Print and shaded views of the part. All mm, measured from the part's lowest x, y and z. A direction names the side the tool comes from. Round coordinates to 2 decimals unless told otherwise and drop trailing zeros. Loops run counter-clockwise (first coordinate to the right, second up) from the corner with the lowest first, then second, coordinate; pieces in that order, holes last. Notation, with made-up numbers: (54, -16.5) -> (105, -16.5) arc R20 ccw to (105, -2.5) -> close; hole circle Ø8 at (-27, 69). An arc over 180 degrees is marked (long way). Answer as CSV lines item,"result".
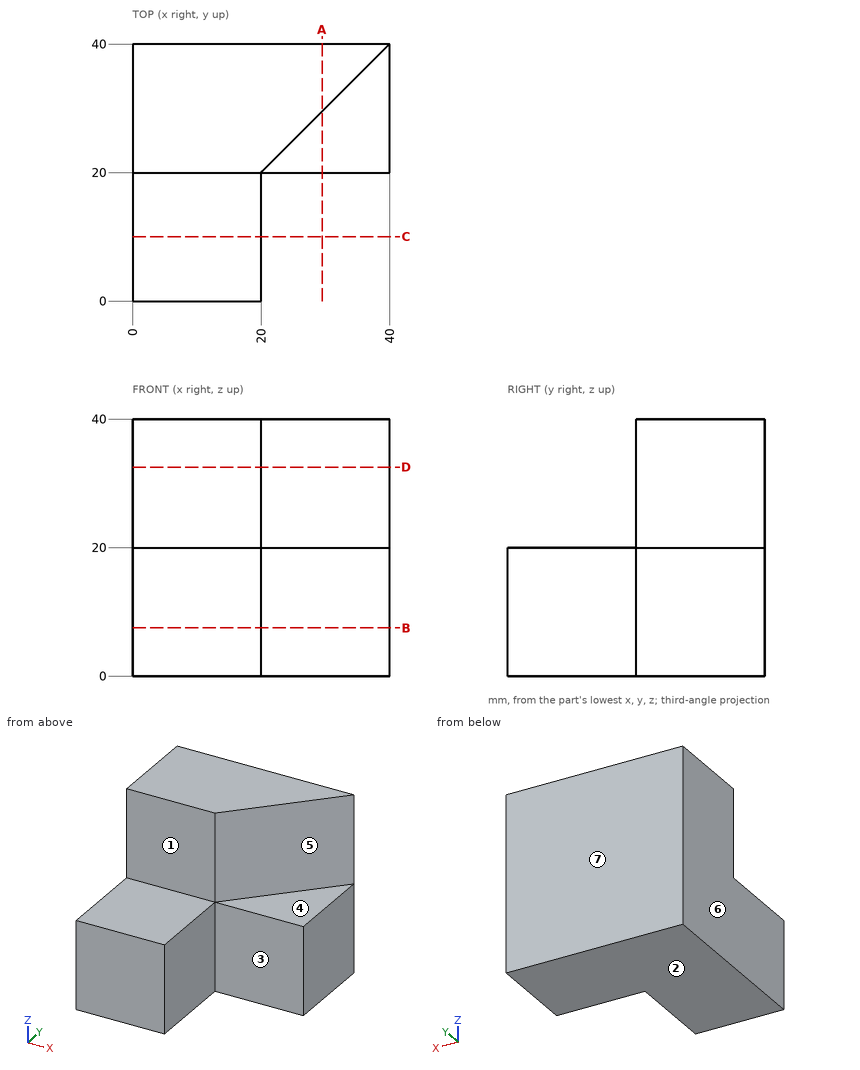
Q1. Saw through at D-D, the plane z = 32.5. Write the cut outline in (x, y).
Geometry results:
outline,"(0, 20) -> (20, 20) -> (40, 40) -> (0, 40) -> close"
Q2. Saw through at C-C, the plane y = 10. Write the cut outline in (x, z).
Geometry results:
outline,"(0, 0) -> (20, 0) -> (20, 20) -> (0, 20) -> close"
Q3. Saw through at A-A, the plane x = 29.5. Write the cut outline in (y, z).
Geometry results:
outline,"(20, 0) -> (40, 0) -> (40, 40) -> (29.5, 40) -> (29.5, 20) -> (20, 20) -> close"
Q4. Which spindle directions (+Z, -Z, +X, -X, +Y, -Y) get a long thin tool onto all of the face, cutting with end or side? Do the marked faces 1, 2, 3 and 4. Say none if no direction does.
Geometry results:
face 1,"+Z, +X, -X, -Y"
face 2,"-Z, +X, -X, +Y, -Y"
face 3,"+Z, -Z, +X, -Y"
face 4,"+Z, +X, -Y"
Q5. Drop flat-ended pins along their axis: P1, Ø10, axis at x = 5.5, z = 34.5, coming from the -Y side; P2, Ø12, axis at y = 22.5, z = 24, coming from the -X side; P3, Ø10, axis at x = 8.5, y = 5, coming from the +Z side; P4, Ø1, axis at y = 17.5, z = 11, coming from the +X side. Give the stop position or say it passes through.
Geometry results:
P1,"y = 20"
P2,"x = 0"
P3,"z = 20"
P4,"x = 20"
Q6. Drill centre lines: line 1 along Z through (x, y) = (16, 11); line 2 along Y through (x, z) = (25.5, 16). Where is each one in solid material? Low to high.
Geometry results:
line 1,"0 to 20"
line 2,"20 to 40"
Q7. Saw through at B-B, the plane z = 7.5. Write the cut outline in (x, y), then the cut area to 3 significant figures.
Geometry results:
outline,"(0, 0) -> (20, 0) -> (20, 20) -> (40, 20) -> (40, 40) -> (0, 40) -> close"
area,"1,200 mm2"
Q8. Two-plate mould, pull along Y, no slides. Class the marked faces 5, 6 and 7: pulls with the +Y half, pulls with the -Y half, needs draft (parallel to the pull), parting line crosses it, or undercut.
Geometry results:
face 5,"pulls with the -Y half"
face 6,"needs draft"
face 7,"pulls with the +Y half"
